Here's the drawing with two shaded views (mm, measured from the low corner). I have some questions. Round coordinates to 2 decimals unless told otherwise and drop trailing zeros. Order: outer loops, then holes, each group sorted by start corner. A loop starts at its lowest first (then second) coordinate and runs counter-clockwise, first axis right, second up.
Q1. Will these pins go through, and if not, where does the flat tip stop? P1, Ø3, axis at y = 11.5, z = 19.5, coming from the -X side; P2, Ø12, axis at x = 12.5, y = 3.5, coming from the +Z side; P3, Ø2, axis at x = 34.5, y = 15.5, coming from the +Z side.
Q2. If we section it at D-D (y = 13): Please give me the cut outline in (x, z), plus the area to 3 significant figures.
Q3. If we section it at C-C (y = 18.5): Please give me the cut outline in (x, z).
Q4. We'd pull the mould along Y, two halves only. Please class the marked faces 1, 2, 3 and 4: pulls with the +Y half, pulls with the -Y half, needs draft (parallel to the pull), parting line crosses it, or undercut.
Q5. If we section it at A-A (z = 20): Please give me the cut outline in (x, y), plus the area to 3 significant figures.
Q6. If I drill on line 1 (Y direction, x = 17.5, z = 34.5); line 2 (Z direction, x = 20, y = 18.4); line 3 (Y direction, x = 8, z = 19.5), over which ranges is the centre line in solid material (lowest first)?
Q7. If we section it at B-B (x = 20): Please give me the cut outline in (y, z).
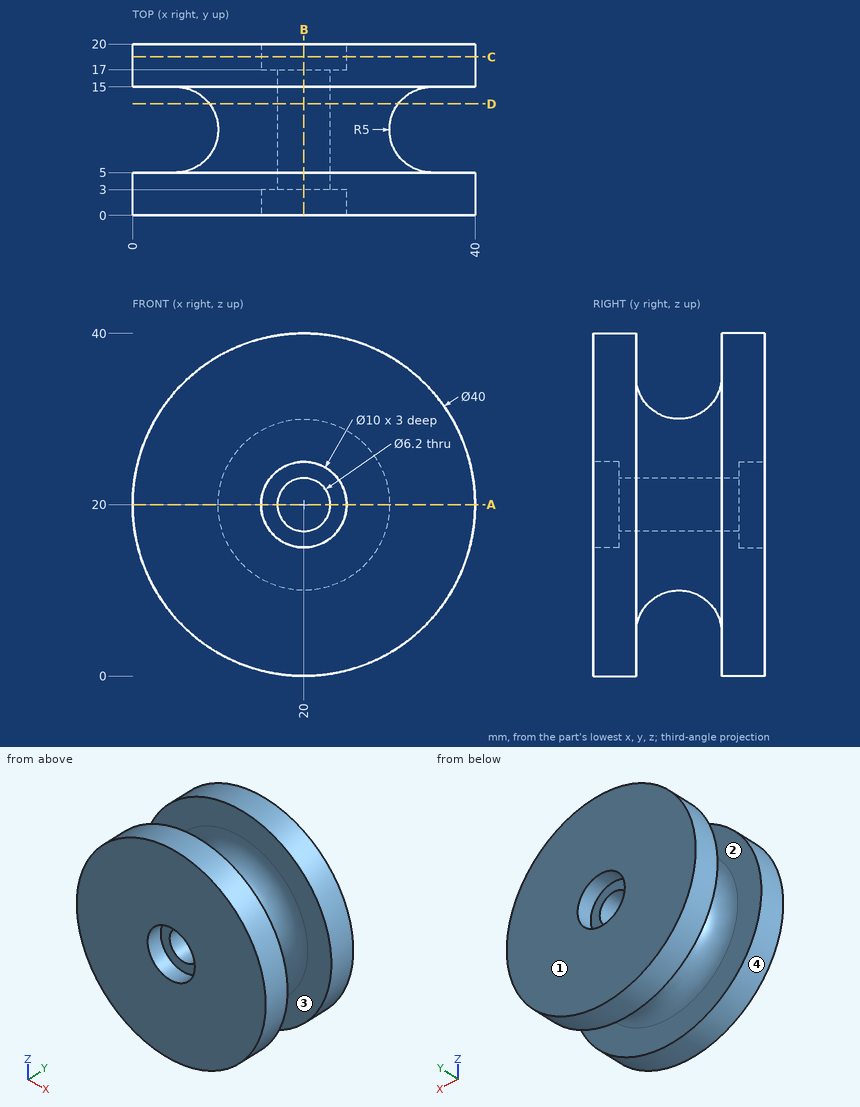
Solution:
1. P1: stops at x = 9.01
1. P2: stops at z = 39.94
1. P3: stops at z = 34.76
2. outline: circle Ø22 at (20, 20); hole circle Ø6.2 at (20, 20)
2. area: 350 mm2
3. outline: circle Ø40 at (20, 20); hole circle Ø10 at (20, 20)
4. face 1: pulls with the +Y half
4. face 2: undercut
4. face 3: undercut
4. face 4: needs draft
5. outline: (0, 0) - (15, 0) - (15, 3) - (16.9, 3) - (16.9, 17) - (15, 17) - (15, 20) - (0, 20) - (0, 15) - (5, 15) arc R5 cw to (5, 5) - (0, 5) - close; (23.1, 3) - (25, 3) - (25, 0) - (40, 0) - (40, 5) - (35, 5) arc R5 cw to (35, 15) - (40, 15) - (40, 20) - (25, 20) - (25, 17) - (23.1, 17) - close
5. area: 475 mm2
6. line 1: y = 0 to 5.01, 14.99 to 20
6. line 2: z = 0 to 15, 25 to 40
6. line 3: y = 0 to 5.99, 14.01 to 20
7. outline: (0, 0) - (5, 0) - (5, 5) arc R5 cw to (15, 5) - (15, 0) - (20, 0) - (20, 15) - (17, 15) - (17, 16.9) - (3, 16.9) - (3, 15) - (0, 15) - close; (0, 25) - (3, 25) - (3, 23.1) - (17, 23.1) - (17, 25) - (20, 25) - (20, 40) - (15, 40) - (15, 35) arc R5 cw to (5, 35) - (5, 40) - (0, 40) - close
